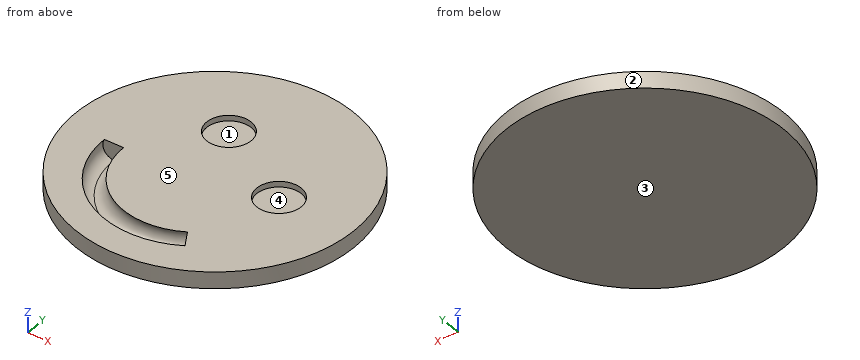
```python
from build123d import *

# Parameters (mm, degrees)
CYLINDER001_R          = 4
CYLINDER001_DEPTH      = 2
CYLINDER002_R          = 4
CYLINDER002_DEPTH      = 2
FUSION_PLACEMENT_ANGLE = 30
TORUS_R                = 2
TORUS_ANGLE            = 120
CYLINDER_R             = 25
CYLINDER_DEPTH         = 3


with BuildPart() as ull1:
    # Cylinder001 → Cylinder001 (new body)
    with BuildSketch(Plane(origin=(9, 9, 2), x_dir=(1, 0, 0), z_dir=(0, 0, 1))):
        Circle(CYLINDER001_R)
    extrude(amount=CYLINDER001_DEPTH)


with BuildPart() as fusion:
    # Cylinder002 → Cylinder002 (new body)
    with BuildSketch(Plane(origin=(-9, 9, 2), x_dir=(1, 0, 0), z_dir=(0, 0, 1))):
        Circle(CYLINDER002_R)
    extrude(amount=CYLINDER002_DEPTH)

    # Fusion: union ull1
    add(ull1.part)


with BuildPart() as fusion_1:
    # Fusion placement: moved
    add(fusion.part.moved(Location((-1, -3, 0))).rotate(Axis((-1, -3, 0), (0, 0, -1)), FUSION_PLACEMENT_ANGLE))


with BuildPart() as torus:
    # Torus → Torus (revolve)
    with BuildSketch(Plane(origin=(-1, -3, 2), x_dir=(-1, 0, 0), z_dir=(0, 1, 0))):
        with Locations((15, 0)):
            Circle(TORUS_R)
    revolve(axis=Axis((-1, -3, 2), (0, 0, 1)), revolution_arc=TORUS_ANGLE)


with BuildPart() as cut001:
    # Cylinder → Cylinder (new body)
    with BuildSketch(Plane.XY):
        Circle(CYLINDER_R)
    extrude(amount=CYLINDER_DEPTH)

    # Cut: cut Torus
    add(torus.part, mode=Mode.SUBTRACT)

    # Cut001: cut Fusion
    add(fusion_1.part, mode=Mode.SUBTRACT)


solid = cut001.part
```
Model file for the job. Use its own axes, mm. Face numbers are marked on the shaded views. A direction names the side the tool comes from. Coordinates: 2 decimals unless noted, no trailing zeros. Loops run counter-clockwise (first coordinate to the right, second up) from the corner with the lowest first, then second, coordinate; pieces in that order, holes last. Notation, with made-up numbers: (3, 80) -> (14, 80) arc R15 cw to (14, 109) -> close; hole circle Ø1 at (50.5, 0.5). An arc over 180 degrees is marked (long way). Answer as a JSON object with one key per item and string values.
Q1. Cut at C-C (y = 21). List the corners of the cut face in (x, z), and give its area (3 significant figures).
Report:
{"outline": "(-13.56, 0) -> (13.56, 0) -> (13.56, 3) -> (-13.56, 3) -> close", "area": "81.4 mm2"}
Q2. Cut at B-B (y = 0). List the corners of the cut face in (x, z), and give its area (3 significant figures).
Report:
{"outline": "(-25, 0) -> (25, 0) -> (25, 3) -> (15.28, 3) -> (15.28, 2) -> (7.31, 2) -> (7.31, 3) -> (-25, 3) -> close", "area": "142 mm2"}
Q3. Flat gauge pins, fed straight in: P1, Ø1, axis at y = -18.5, z = 1.5, coming from the +X side; P2, Ø7, axis at x = 11.29, y = 0.29, coming from the +Z side. Where does each tip first touch, or does it go through?
Report:
{"P1": "stops at x = 17.35", "P2": "stops at z = 2"}
Q4. Probe probe 1 along Y at (x, z) = (-5, 2.15); probe 2 along X at (y, z) = (-10, 2.25); probe 3 along Y at (x, z) = (13, 2.1). List the from-to ranges inside material, lowest first.
Report:
{"probe 1": "y = -24.49 to -19.52, -15.38 to 5.36, 13.23 to 24.49", "probe 2": "x = -22.91 to -16.47, -11.97 to 22.91", "probe 3": "y = -21.35 to -3.32, 3.91 to 21.35"}
Q5. Cut at A-A (z = 1.45). List the corners of the cut face in (x, y).
Report:
{"outline": "circle Ø50 at (0, 0); hole (-17.92, -3) arc R16.92 ccw to (7.46, -17.66) -> (5.54, -14.33) arc R13.08 cw to (-14.08, -3) -> close"}
Q6. 3-axis set-ups, long thin cutter, end or side, ignore diameter. For the marked faces 4 and 5: which of +Z, -Z, +X, -X, +Y, -Y reach the whole face in a straight line?
Report:
{"face 4": "+Z", "face 5": "+Z, +X, -X, +Y, -Y"}
Q7. Pull direction Y, two halves, no side cores. Call the marked faces 1, 2 and 3: released by +Y, released by -Y, zero draft, split by the parting line, or undercut.
Report:
{"face 1": "undercut", "face 2": "split by the parting line", "face 3": "zero draft"}
